```python
from build123d import *

# Parameters (mm, degrees)
EXTRUDE_2_DEPTH     = 12
CHAMFER_1_SIZE      = 2
SKETCH_4_R          = 3
CUT_EXTRUDE_4_DEPTH = 29.861739379


with BuildPart() as part:
    # Эскиз2 → Вытянуть2 (new body)
    with BuildSketch(Plane.XY):
        Polygon((0.846446281, 0), (-29.153553719, 0), (-29.153553719, 4.760108812), (-19.153553719, 4.760108812), (-19.153553719, 17), (-9.153553719, 17), (-9.153553719, 4.760108812), (0.846446281, 4.760108812), align=None)
    extrude(amount=EXTRUDE_2_DEPTH)

    # Фаска1
    chamfer_1_edges = [part.edges().sort_by_distance(p)[0] for p in [
        (-14.153553719, 17, 12),
        (-14.153553719, 17, 0),
    ]]
    chamfer(chamfer_1_edges, length=CHAMFER_1_SIZE)

    # Эскиз4 → Вытянуть4 (cut, through all)
    with BuildSketch(Plane.ZY.offset(19.153553719)):
        with Locations((6, 12.217021039)):
            Circle(SKETCH_4_R)
    extrude(amount=-CUT_EXTRUDE_4_DEPTH, mode=Mode.SUBTRACT)


solid = part.part
```
The model under review builds one solid part; all positions refer to its coordinate system, in mm. A direction names the side the tool comes from. Give positions to 0.01 mm unless a question says otherwise; leave off trailing zeros. Write each loop counter-clockwise with the first axis right and the second up, starting at its lowest first coordinate (ties: lowest second). Pieces come first, ordered by that corner, then holes. Notation, with made-up numbers: M 24.25,58.25 L 44.25,58.25 A15 ccw 44.25,66.25 Z; hole C -5,-4 d6. An arc over 180 degrees is marked long. Answer in a Markdown table with one row per item.
Item 1: Add section A-A on z = 6. Give the boundary of the cut face in (x, y), plus the area to 3 significant figures.
Check sheet entries:
| item | result |
|---|---|
| outline | M -29.15,0 L 0.85,0 L 0.85,4.76 L -9.15,4.76 L -9.15,9.22 L -19.15,9.22 L -19.15,4.76 L -29.15,4.76 Z; M -19.15,15.22 L -9.15,15.22 L -9.15,17 L -19.15,17 Z |
| area | 205 mm2 |
Item 2: For P1, Ø5, axis at x = -9.5, z = 1, coming from the +Y side; P2, Ø3, axis at x = -4.5, z = 5.5, coming from the +Y side; P3, Ø6, axis at y = 9, z = 3.5, coming from the +X side, all flat-tipped, find the tip position at first contact; note any pin that passes through.
Check sheet entries:
| item | result |
|---|---|
| P1 | y = 17 |
| P2 | y = 4.76 |
| P3 | x = -9.15 |
Item 3: For line 1 along Z through (x, y) = (-13.5, 12); line 2 along Y through (x, z) = (-13, 6); line 3 along X through (y, z) = (9.75, 11.5), list the stretches that pass through material, from the lowest coordinate up.
Check sheet entries:
| item | result |
|---|---|
| line 1 | 0 to 3.01, 8.99 to 12 |
| line 2 | 0 to 9.22, 15.22 to 17 |
| line 3 | -19.15 to -9.15 |
Item 4: Add section B-B on y = 11.5. Give the boundary of the cut face in (x, z).
Check sheet entries:
| item | result |
|---|---|
| outline | M -19.15,0 L -9.15,0 L -9.15,3.09 L -19.15,3.09 Z; M -19.15,8.91 L -9.15,8.91 L -9.15,12 L -19.15,12 Z |
Item 5: Tool access review of faces 1 (the face through (-4, 4.76, 6)), 2 (the face through (-24, 4.76, 6)), 3 (the face through (-29.154, 2, 6)): name each direction out of +Z, -Z, +X, -X, +Y, -Y from which nothing blocks a thin tool from reaching the whole face with its end or side.
Check sheet entries:
| item | result |
|---|---|
| face 1 | +Z, -Z, +X, +Y |
| face 2 | +Z, -Z, -X, +Y |
| face 3 | +Z, -Z, -X, +Y, -Y |
Item 6: Add section D-D on x = -8.5. Give the boundary of the cut face in (y, z).
Check sheet entries:
| item | result |
|---|---|
| outline | M 0,0 L 4.76,0 L 4.76,12 L 0,12 Z |
Item 7: Draft analysis for pull direction Z (two halves, no side actions). For faces 4 (the face through (-14, 6, 12)), 5 (the face through (-19.154, 9, 5)), 6 (the face through (-14.224, 9.556, 7.384)), 7 (the face through (-14, 6, 0)), state which applies: +Z half, -Z half, draft (parallel to the pull), parting line (faces both ways), or undercut.
Check sheet entries:
| item | result |
|---|---|
| face 4 | +Z half |
| face 5 | draft |
| face 6 | undercut |
| face 7 | -Z half |
Item 8: Add section C-C on x = -17.5. Give the boundary of the cut face in (y, z), plus the area to 3 significant figures.
Check sheet entries:
| item | result |
|---|---|
| outline | M 0,0 L 15,0 L 17,2 L 17,10 L 15,12 L 0,12 Z; hole C 12.22,6 d6 |
| area | 172 mm2 |
